from build123d import *

# Parameters (mm, degrees)
F0_W     = 24
F0_H     = 3
F0_W_2   = 48
F0_H_2   = 5
F0_W_3   = 13
F0_W_4   = 5
F0_W_5   = 10
F0_W_6   = 5.462219
F0_W_7   = 8
F2_DEPTH = 5


with BuildPart() as f2:
    # F0 (on Front) → F2 (new body)
    with BuildSketch(Plane.XZ):
        Polygon((-44.148275, 55), (-55.860446, 55), (-55.860446, 45), (-38.860446, 45), (-38.860446, 40), (-55.860446, 40), (-55.860446, 25), (-38.860446, 25), (-38.860446, 20), (-55.860446, 20), (-55.860446, 5), (-38.860446, 5), (-38.860446, 0), (-55.860446, 0), (-55.860446, -15), (-38.860446, -15), (-38.860446, -20), (-55.860446, -20), (-55.860446, -32.565833), (-38.860446, -32.565833), (-38.860446, -37.565833), (-55.860446, -37.565833), (-55.860446, -51.917288), (-38.860446, -51.917288), (-38.860446, -56.917288), (-55.860446, -56.917288), (-55.860446, -63.862034), (-47.860446, -63.862034), (-30.842662, -63.862034), (-20.842662, -63.862034), (-16.148275, -63.862034), (-10.686056, -63.862034), (2.313944, -63.862034), (10.461201, -63.862034), (10.461201, -56.917288), (-6.538799, -56.917288), (-6.538799, -51.917288), (10.461201, -51.917288), (10.461201, -37.565833), (-6.538799, -37.565833), (-6.538799, -32.565833), (10.461201, -32.565833), (10.461201, -20), (-6.538799, -20), (-6.538799, -15), (10.461201, -15), (10.461201, 0), (-6.538799, 0), (-6.538799, 5), (10.461201, 5), (10.461201, 20), (-6.538799, 20), (-6.538799, 25), (10.461201, 25), (10.461201, 40), (-6.538799, 40), (-6.538799, 45), (10.461201, 45), (10.461201, 55), (6.173372, 55), (-6.826628, 55), (-16.148275, 55), (-21.148275, 55), (-31.148275, 55), align=None)
        with Locations((-22.360446, -54.425548)):
            Rectangle(F0_W, F0_H, mode=Mode.SUBTRACT)
        with Locations((-20.532146, -45.065833)):
            Rectangle(F0_W_2, F0_H_2, mode=Mode.SUBTRACT)
        with Locations((-22.360446, -35.106815)):
            Rectangle(F0_W, F0_H, mode=Mode.SUBTRACT)
        with Locations((-21.860446, -25.065833)):
            Rectangle(F0_W_2, F0_H_2, mode=Mode.SUBTRACT)
        with Locations((-22.360446, -17.415623)):
            Rectangle(F0_W, F0_H, mode=Mode.SUBTRACT)
        with Locations((-21.860446, -7.5)):
            Rectangle(F0_W_2, F0_H_2, mode=Mode.SUBTRACT)
        with Locations((-22.360446, 2.570768)):
            Rectangle(F0_W, F0_H, mode=Mode.SUBTRACT)
        with Locations((-21.860446, 12.5)):
            Rectangle(F0_W_2, F0_H_2, mode=Mode.SUBTRACT)
        with Locations((-22.360446, 22.768489)):
            Rectangle(F0_W, F0_H, mode=Mode.SUBTRACT)
        with Locations((-21.860446, 32.5)):
            Rectangle(F0_W_2, F0_H_2, mode=Mode.SUBTRACT)
        with Locations((-22.360446, 42.321008)):
            Rectangle(F0_W, F0_H, mode=Mode.SUBTRACT)
        with Locations((-22.360446, 50.378293)):
            Rectangle(F0_W, F0_H, mode=Mode.SUBTRACT)
        with Locations((-37.648275, 57.5)):
            Rectangle(F0_W_3, F0_H_2)
        with Locations((-18.648275, 57.5)):
            Rectangle(F0_W_4, F0_H_2)
        with Locations((-0.326628, 57.5)):
            Rectangle(F0_W_3, F0_H_2)
        with Locations((-25.842662, -66.362034)):
            Rectangle(F0_W_5, F0_H_2)
        with Locations((-13.417165, -66.362034)):
            Rectangle(F0_W_6, F0_H_2)
        Polygon((10.461201, -63.862034), (2.313944, -63.862034), (2.313944, -68.862034), (10.313944, -68.862034), align=None)
        with Locations((-51.860446, -66.362034)):
            Rectangle(F0_W_7, F0_H_2)
    extrude(amount=F2_DEPTH)


solid = f2.part
The listing builds one solid part. Answer for the finished solid, in the listing's coordinates (mm). A direction names the side the tool comes from. Give positions to 0.01 mm unless a question says otherwise; leave off trailing zeros. Loops run counter-clockwise (first coordinate to the right, second up) from the corner with the lowest first, then second, coordinate; pieces in that order, holes last. Notation, with made-up numbers: (84, 49.25) - (96, 49.25) arc R24 cw to (96, 79.25) - close; hole circle Ø9 at (-30.5, -11). An arc over 180 degrees is marked (long way). Use one line per item in the form item = value.
1. Section A-A on x = 5 is taken. Give the vertices of the cut face in (y, z), then the cut area to 3 significant figures.
Calculated:
outline = (-5, -68.86) - (0, -68.86) - (0, -56.92) - (-5, -56.92) - close; (-5, -51.92) - (0, -51.92) - (0, -37.57) - (-5, -37.57) - close; (-5, -32.57) - (0, -32.57) - (0, -20) - (-5, -20) - close; (-5, -15) - (0, -15) - (0, 0) - (-5, 0) - close; (-5, 5) - (0, 5) - (0, 20) - (-5, 20) - close; (-5, 25) - (0, 25) - (0, 40) - (-5, 40) - close; (-5, 45) - (0, 45) - (0, 60) - (-5, 60) - close
area = 494 mm^2
2. Section B-B on x = -36 is taken. Give the vertices of the cut face in (y, z), then the cut area to 3 significant figures.
Calculated:
outline = (-5, -63.86) - (0, -63.86) - (0, -47.57) - (-5, -47.57) - close; (-5, -42.57) - (0, -42.57) - (0, -27.57) - (-5, -27.57) - close; (-5, -22.57) - (0, -22.57) - (0, -10) - (-5, -10) - close; (-5, -5) - (0, -5) - (0, 10) - (-5, 10) - close; (-5, 15) - (0, 15) - (0, 30) - (-5, 30) - close; (-5, 35) - (0, 35) - (0, 60) - (-5, 60) - close
area = 494 mm^2
3. Given pin 1 Ø1.5 at (x, y) = (-18, -2) entering from -Z; pin 2 Ø1.5 at (x, y) = (-50.5, -2.5) entering from +Z; pin 3 Ø2.5 at (y, z) = (-1.5, 23) entering from +X, each flat-ended and moving along its own axis, determine where each tip first touches the part or whether it passes through.
Calculated:
pin_1 = -63.86
pin_2 = 55
pin_3 = -6.54
4. Section C-C on y = -2.05 is taken. Count the separate pieces of the cut face and the enclosed holes in it, then the cut area to 3 significant figures.
Calculated:
separate_pieces = 1
enclosed_holes = 12
area = 5,470 mm^2
5. Which of the six approach directions +Z, -Z, +X, -X, +Y, -Y give full straight-line access (tool end or side, diameter ignored) to faces 4 (the face through (2, -2, -37.566)), 5 (the face through (-47, -2, -15)), 6 (the face through (-55.86, -2, -26)), 7 (the face through (2.14, -2, 32))?
Calculated:
face_4 = +X, +Y, -Y
face_5 = -X, +Y, -Y
face_6 = +Z, -Z, -X, +Y, -Y
face_7 = +Y, -Y
6. Find the intervals of material crossed by line 1 along X through (y, z) = (-3.4, -45); line 2 along Z through (x, y) = (-35.5, -2.3); line 3 along X through (y, z) = (-1.8, -53.5), in increasing order. Write a range as [from, to].
Calculated:
line_1 = [-55.86, -44.53], [3.47, 10.46]
line_2 = [-63.86, -47.57], [-42.57, -27.57], [-22.57, -10], [-5, 10], [15, 30], [35, 60]
line_3 = [-38.86, -34.36], [-10.36, -6.54]
7. The mould has two halves that part along X. Classify faces 1 (the face through (-47, -2, 0)), 2 (the face through (-38.86, -2, 43)), 3 (the face through (-34.36, -2, -17)): pulls with the +X half, pulls with the -X half, needs draft (parallel to the pull), parting line crosses it, or undercut.
Calculated:
face_1 = needs draft
face_2 = pulls with the -X half
face_3 = undercut
